Build history of the part. All positions in model axes, mm. A direction names the side the tool comes from. Round coordinates to 2 decimals unless told otherwise and drop trailing zeros. Write each loop counter-clockwise with the first axis right and the second up, starting at its lowest first coordinate (ties: lowest second). Pieces come first, ordered by that corner, then holes. Notation, with made-up numbers: M 64.25,40.5 L 88.25,40.5 A13 ccw 88.25,44.5 Z; hole C 11,-22 d3. An arc over 180 degrees is marked long. Write item = value, one per line. Start each with the question number.
Q1. Probe L1, parallel to X at y = 6, z = -50; L2, parallel to X at y = 17, z = -66; L3, parallel to Y at x = 38.5, z = -62. List the from-to ranges inside material, lowest first.
Q2. Band-saw the part on A-A on y = 26. Write the cut outline in (x, z), plus the area to 3 significant figures.
Q3. Drop flat-ended pins along their axis: P1, Ø5, axis at x = 2, y = 14.5, coming from the +Z side; P2, Ø12, axis at y = 24.5, z = 45.5, coming from the +X side; P3, Ø8, axis at y = 19, z = -16, coming from the +X side; P4, Ø1, axis at x = -79, z = 38.5, coming from the +Y side. Give the stop position or say it passes through.
Q4. Pull direction X, two halves, no side cores. Call faces 1 (the flat face through (41, 20, -5)), 2 (the cylindrical face through (5.016, 25.21, 15.929)), 3 (the flat face through (-69.2, 15, 0)): released by +X, released by -X, zero draft, split by the parting line, or undercut.
Q5. Tool access for faces 4 (the cylindrical face through (-8.618, 24.79, 20.784)), 5 (the flat face through (41, 20, 5)), 6 (the flat face through (-41, 20, 5)), 7 (the flat face through (-41, 20, -5)): list every direction of +Z, -Z, +X, -X, +Y, -Y with a clear straight run to the whole face (end or side of a thin tool).
Q6. Band-saw the part on C-C on x = -36. Write the cut outline in (y, z).
Q7. Band-saw the part on B-B on z = -50. Write the cut outline in (x, y).
Q8. Band-saw the part on D-D on z = 40. Write the cut outline in (x, y), plus the area to 3 significant figures.
```python
from build123d import *

# Parameters (mm, degrees)
CROQUIS1_R              = 22.5
SALIENTE_EXTRUIR1_DEPTH = 40
CROQUIS2_R              = 16.7
CROQUIS2_R_2            = 13.3
CORTAR_EXTRUIR1_DEPTH   = 30
SALIENTE_EXTRUIR2_DEPTH = 10
SALIENTE_EXTRUIR5_DEPTH = 5
MATRIZC1_COUNT          = 4
CROQUIS5_R              = 4.25
CORTAR_EXTRUIR2_DEPTH   = 136.646599663


with BuildPart() as part:
    # Croquis1 → Saliente-Extruir1 (new body)
    with BuildSketch(Plane(origin=(0, 0, 0), x_dir=(1, 0, 0), z_dir=(0, 1, 0))):
        with Locations(Location((0, 0, 0), (0, 0, 270))):
            Circle(CROQUIS1_R)
    extrude(amount=SALIENTE_EXTRUIR1_DEPTH)

    # Croquis2 → Cortar-Extruir1 (cut)
    with BuildSketch(Plane(origin=(0, 40, 0), x_dir=(1, 0, 0), z_dir=(0, 1, 0))):
        with Locations(Location((0, 0, 0), (0, 0, 270))):
            Circle(CROQUIS2_R)
        with Locations(Location((0, 0, 0), (0, 0, 270))):
            Circle(CROQUIS2_R_2, mode=Mode.SUBTRACT)
    extrude(amount=-CORTAR_EXTRUIR1_DEPTH, mode=Mode.SUBTRACT)

    # Croquis3 → Saliente-Extruir2 (add)
    with BuildSketch(Plane.XZ):
        Polygon((50, 86.602540378), (-50, 86.602540378), (-100, 0), (-50, -86.602540378), (50, -86.602540378), (100, 0), align=None)
    extrude(amount=-SALIENTE_EXTRUIR2_DEPTH)

    # Croquis4 → Saliente-Extruir5 (add, symmetric)
    with BuildSketch(Plane(origin=(0, 0, 0), x_dir=(0, 0, -1), z_dir=(1, 0, 0))):
        Polygon((-69.2, 10), (-19.2, 10), (-19.2, 35), (-69.2, 20), align=None)
    saliente_extruir5 = extrude(amount=SALIENTE_EXTRUIR5_DEPTH, both=True)

    # MatrizC1: Saliente-Extruir5 ×4 about axis
    matrizc1_axis = Axis((0, 0, 0), (0, 1, 0))
    for i in range(1, MATRIZC1_COUNT):
        add(saliente_extruir5.rotate(matrizc1_axis, i * 360 / MATRIZC1_COUNT))

    # Croquis5 → Cortar-Extruir2 (cut, through all)
    with BuildSketch(Plane(origin=(0, 10, 0), x_dir=(1, 0, 0), z_dir=(0, 1, 0))):
        with Locations(Location((-50, 50, 0), (0, 0, 270))):
            Circle(CROQUIS5_R)
        with Locations(Location((50, 50, 0), (0, 0, 270))):
            Circle(CROQUIS5_R)
        with Locations(Location((-50, -50, 0), (0, 0, 270))):
            Circle(CROQUIS5_R)
        with Locations(Location((50, -50, 0), (0, 0, 270))):
            Circle(CROQUIS5_R)
    extrude(amount=-CORTAR_EXTRUIR2_DEPTH, mode=Mode.SUBTRACT)


solid = part.part
```
Conclusion:
q1.L1 = -71.13 to -54.25, -45.75 to 45.75, 54.25 to 71.13
q1.L2 = -5 to 5
q1.L3 = 0 to 10
q2.outline = M -49.2,-5 L -21.94,-5 A22.5 ccw -5,-21.94 L -5,-49.2 L 5,-49.2 L 5,-21.94 A22.5 ccw 21.94,-5 L 49.2,-5 L 49.2,5 L 21.94,5 A22.5 ccw 5,21.94 L 5,49.2 L -5,49.2 L -5,21.94 A22.5 ccw -21.94,5 L -49.2,5 Z; C 0,0 d26.6; hole C 0,0 d33.4
q2.area = 2,350 mm^2
q3.P1 = 69.2
q3.P2 = 5
q3.P3 = 19.03
q3.P4 = through
q4.face_1 = zero draft
q4.face_2 = undercut
q4.face_3 = released by -X
q5.face_4 = +Y
q5.face_5 = +Z, +X, +Y
q5.face_6 = +Z, -X, +Y
q5.face_7 = -Z, -X, +Y
q6.outline = M 0,-86.6 L 10,-86.6 L 10,-5 L 29.96,-5 L 29.96,5 L 10,5 L 10,86.6 L 0,86.6 Z
q7.outline = M -71.13,0 L -54.25,0 L -54.25,10 L -71.13,10 Z; M -45.75,0 L 45.75,0 L 45.75,10 L 5,10 L 5,25.76 L -5,25.76 L -5,10 L -45.75,10 Z; M 54.25,0 L 71.13,0 L 71.13,10 L 54.25,10 Z
q8.outline = M -76.91,0 L 76.91,0 L 76.91,10 L 5,10 L 5,28.76 L -5,28.76 L -5,10 L -76.91,10 Z
q8.area = 1,730 mm^2
